Work out the finished part from the listing and answer in its coordinate system (mm). A direction names the side the tool comes from. Give positions to 0.01 mm unless a question says otherwise; leave off trailing zeros. Loops run counter-clockwise (first coordinate to the right, second up) from the corner with the lowest first, then second, coordinate; pieces in that order, holes last. Notation, with made-up numbers: M 88,84 L 96,84 A19 ccw 96,107 Z; hole C 79,27.25 d10. An arc over 180 degrees is marked long. Use a Markdown table: item, result.
```python
from build123d import *

# Parameters (mm, degrees)
F0_W     = 152.4
F0_H     = 76.2
F0_R     = 12.7
F1_DEPTH = 25.4
F2_T     = -2.54
F4_D     = 6.35


with BuildPart() as f1:
    # F0 (on Front) → F1 (new body)
    with BuildSketch(Plane.XZ):
        Rectangle(F0_W, F0_H)
        with Locations((38.1, 0)):
            Circle(F0_R, mode=Mode.SUBTRACT)
    extrude(amount=F1_DEPTH)

    # F2
    f2_openings = [f1.faces().sort_by_distance(p)[0] for p in [
        (-1.738273, -25.4, 0),
    ]]
    offset(amount=F2_T, openings=f2_openings)

    # F4 (through all)
    with Locations(Plane(origin=(0, 0, 0), x_dir=(1, 0, 0), z_dir=(0, 1, 0))):
        with Locations((-49.7758053243, -14.3796773627)):
            Hole(F4_D / 2)


solid = f1.part
```
(1) A cutting plane is placed at D-D (z = -18.5). Write down the section's boundary in (x, y).
Entries:
| item | result |
|---|---|
| outline | M -76.2,-25.4 L -73.66,-25.4 L -73.66,-2.54 L 73.66,-2.54 L 73.66,-25.4 L 76.2,-25.4 L 76.2,0 L -76.2,0 Z |
(2) A cutting plane is placed at B-B (z = 0). Write down the section's boundary in (x, y), and give its area (3 significant figures).
Entries:
| item | result |
|---|---|
| outline | M -76.2,-25.4 L -73.66,-25.4 L -73.66,-2.54 L 22.86,-2.54 L 22.86,-25.4 L 25.4,-25.4 L 25.4,0 L -76.2,0 Z; M 50.8,-25.4 L 53.34,-25.4 L 53.34,-2.54 L 73.66,-2.54 L 73.66,-25.4 L 76.2,-25.4 L 76.2,0 L 50.8,0 Z |
| area | 555 mm² |
(3) A cutting plane is placed at A-A (y = -4.25). Write down the section's boundary in (x, z).
Entries:
| item | result |
|---|---|
| outline | M -76.2,-38.1 L 76.2,-38.1 L 76.2,38.1 L -76.2,38.1 Z; C 38.1,0 d30.48; hole M -73.66,-35.56 L 73.66,-35.56 L 73.66,35.56 L -73.66,35.56 Z; hole C 38.1,0 d25.4 |
(4) A cutting plane is placed at C-C (x = 38.1). Write down the section's boundary in (y, z).
Entries:
| item | result |
|---|---|
| outline | M -25.4,-38.1 L 0,-38.1 L 0,-12.7 L -25.4,-12.7 L -25.4,-15.24 L -2.54,-15.24 L -2.54,-35.56 L -25.4,-35.56 Z; M -25.4,12.7 L 0,12.7 L 0,38.1 L -25.4,38.1 L -25.4,35.56 L -2.54,35.56 L -2.54,15.24 L -25.4,15.24 Z |
(5) Consider probe 1 along Z at (x, y) = (38.1, -11.25); probe 2 along Z at (x, y) = (-56, -8.75); probe 3 along X at (y, z) = (-22, 33.5). Determine where each line is inside the solid, lowest interval first. Write a range as [from, to].
Entries:
| item | result |
|---|---|
| probe 1 | z = [-38.1, -35.56], [-15.24, -12.7], [12.7, 15.24], [35.56, 38.1] |
| probe 2 | z = [-38.1, -35.56], [35.56, 38.1] |
| probe 3 | x = [-76.2, -73.66], [73.66, 76.2] |
(6) The mould has two halves that part along X. Classify faces 1 (the flat face through (76.2, -13, -1)), 2 (the flat face through (-1, -13, 38.1)), 3 (the flat face through (73.66, -14, 0)): released by +X, released by -X, zero draft, split by the parting line, or undercut.
Entries:
| item | result |
|---|---|
| face 1 | released by +X |
| face 2 | zero draft |
| face 3 | undercut |
(7) Given P1, Ø1.5, axis at x = 53, z = 13.5, coming from the -Y side; P2, Ø15, axis at x = 38.1, z = 0, coming from the -Y side, each flat-ended and moving along its own axis, determine where each tip first touches the part or whether it passes through.
Entries:
| item | result |
|---|---|
| P1 | stops at y = -2.54 |
| P2 | passes through |
(8) Which of the six approach directions +Z, -Z, +X, -X, +Y, -Y give full straight-line access (tool end or side, diameter ignored) to faces 4 (the flat face through (-1, -14, -35.56)), 5 (the cylindrical face through (-47.44, -1.29, 12.23))?
Entries:
| item | result |
|---|---|
| face 4 | -Y |
| face 5 | +Y, -Y |
